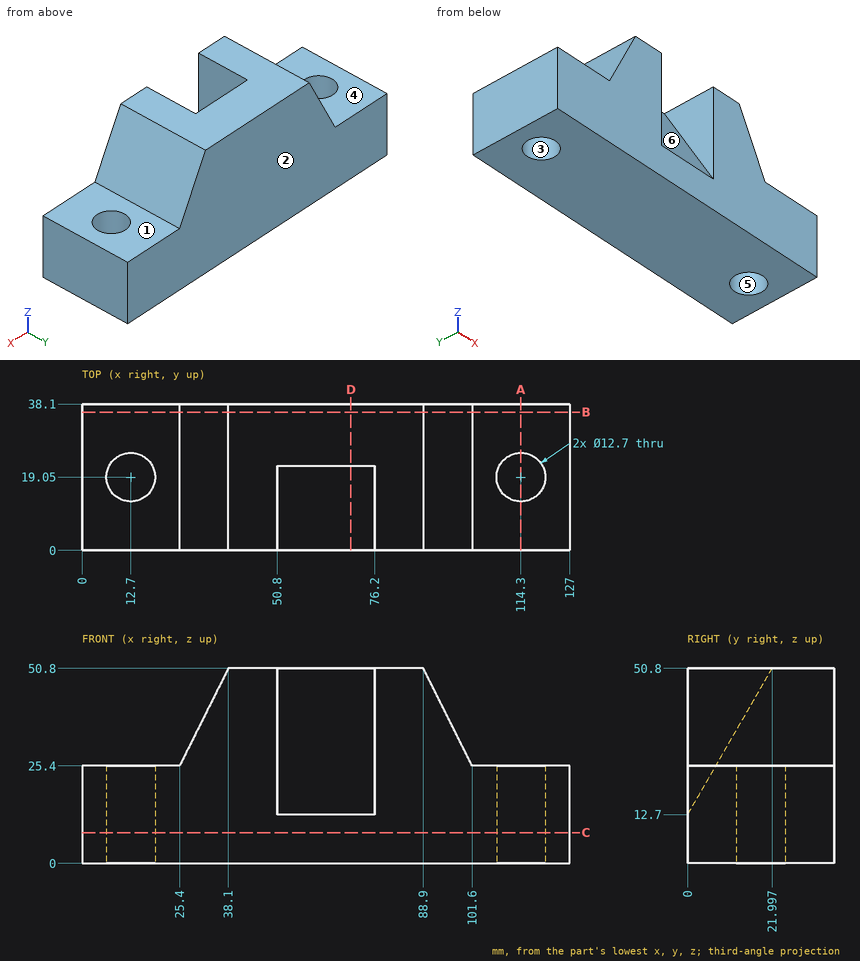
The drawing under review shows one solid part. Ordinate dimensions are in mm from its lowest x, y, z. A direction names the side the tool comes from. Coordinates: 2 decimals unless noted, no trailing zeros. Order: outer loops, then holes, each group sorted by start corner. A loop starts at its lowest first (then second) coordinate and runs counter-clockwise, first axis right, second up. Notation, with made-up numbers: (8.5, -1.5) -> (38.5, -1.5) arc R27 cw to (38.5, 24.5) -> close; hole circle Ø5 at (26, 37.25). An arc over 180 degrees is marked (long way). Answer in a Markdown table with one row per item. Add a question column.
Item 1: Clearance check with flat-ended pins moving along their axes: pin 1 (17.5 mm diameter, centred on y = 9, z = 26.5, fed in from -X); pin 2 (1 mm diameter, centred on y = 12.5, z = 35, fed in from -X); pin 3 (6.5 mm diameter, centred on y = 7, z = 31, fed in from +X) (3 decimals); pin 4 (10 mm diameter, centred on x = 112, y = 25, fed in from +Z). State where each tip first meets the part, or that it passes through.
Item 2: We need section A-A on x = 114.3. Write out the cut boundary in (y, z), plus the area to 3 significant figures.
Item 3: To check wall thickness, follow probe 1 along X at (y, z) = (19, 9); probe 2 along Y at (x, z) = (12.7, 7.5); probe 3 along Z at (x, y) = (20, 13). State the ranges of each line that lie inside material, in increasing order.
Item 4: We need section D-D on x = 70. Write out the cut boundary in (y, z), plus the area to 3 significant figures.
Item 5: Machinability: for the marked faces 4, 5 and 6, which of the approach directions +Z, -Z, +X, -X, +Y, -Y give a long, thin tool a straight path to every point of the face, cutting with its end or side? Answer none if there is none.
Item 6: We need section B-B on y = 36. Write out the cut boundary in (x, z), plus the area to 3 significant figures.
Item 7: We need section C-C on z = 8. Write out the cut boundary in (x, y).
Item 8: Mouldability with a two-part tool opening along Y and no side actions: class the marked faces 1, 2 and 3 as +Y half, -Y half, draft (parallel to the pull), parting line (faces both ways), or undercut.
Final values:
| question | item | result |
|---|---|---|
| 1 | pin 1 | stops at x = 0 |
| 1 | pin 2 | stops at x = 29.95 |
| 1 | pin 3 | stops at x = 100.425 |
| 1 | pin 4 | stops at z = 25.4 |
| 2 | outline | (0, 0) -> (12.7, 0) -> (12.7, 25.4) -> (0, 25.4) -> close; (25.4, 0) -> (38.1, 0) -> (38.1, 25.4) -> (25.4, 25.4) -> close |
| 2 | area | 645 mm2 |
| 3 | probe 1 | x = 0 to 6.35, 19.05 to 107.95, 120.65 to 127 |
| 3 | probe 2 | y = 0 to 12.7, 25.4 to 38.1 |
| 3 | probe 3 | z = 0 to 25.4 |
| 4 | outline | (0, 0) -> (38.1, 0) -> (38.1, 50.8) -> (22, 50.8) -> (0, 12.7) -> close |
| 4 | area | 1,520 mm2 |
| 5 | face 4 | +Z, -X, +Y, -Y |
| 5 | face 5 | +Z, -Z |
| 5 | face 6 | +Z, -Y |
| 6 | outline | (0, 0) -> (127, 0) -> (127, 25.4) -> (101.6, 25.4) -> (88.9, 50.8) -> (38.1, 50.8) -> (25.4, 25.4) -> (0, 25.4) -> close |
| 6 | area | 4,840 mm2 |
| 7 | outline | (0, 0) -> (127, 0) -> (127, 38.1) -> (0, 38.1) -> close; hole circle Ø12.7 at (12.7, 19.05); hole circle Ø12.7 at (114.3, 19.05) |
| 8 | face 1 | draft |
| 8 | face 2 | +Y half |
| 8 | face 3 | undercut |
